Could you check a few things on this model? Use its own coordinates, in mm. Face numbers are marked on the shaded views. A direction names the side the tool comes from. Give positions to 0.01 mm unless a question says otherwise; leave off trailing zeros. Loops run counter-clockwise (first coordinate to the right, second up) from the corner with the lowest first, then second, coordinate; pieces in that order, holes last. Notation, with made-up numbers: (-26, -35) - (15, -35) arc R6 cw to (15, -25) - close; hole circle Ø7 at (2, -0.5). An arc over 180 degrees is marked (long way). Write each question's results on one line, items separated by ' | '. Start each with the question number.
(1) I need wall thicknesses on line 1 (Y direction, x = -5.5, z = 6); line 2 (Y direction, x = 0, z = 12); line 3 (Z direction, x = 14, y = 1). Which ranges of each line are inside material? Lowest first, please.
(2) For pin 1 (12 mm diameter, centred on x = -6.5, y = 17, fed in from +Z); pin 2 (2.5 mm diameter, centred on x = -2.5, z = 12.5, fed in from +Y); pin 3 (1 mm diameter, centred on y = 1.27, z = 1.905, fed in from +X), each with a flat end and sliding along its axis, tell me the tip position at first contact or that it passes through.
(3) Suppose I cut it at D-D (z = 6.5). Please give me the cut outline in (x, y).
(4) If we mould it in two halves opening along X, with no side actions, what happens to the marked faces 1, 2 and 3? For each: released by +X, released by -X, zero draft, split by the parting line, or undercut.
(5) Suppose I cut it at C-C (y = 15). Please give me the cut outline in (x, z) (3 decimals).
(6) Suppose I cut it at A-A (x = 0). Please give me the cut outline in (y, z) (1 decimal), and give its area (3 significant figures).
(7) On a 3-axis mill with a long thin cutter (end or side, diameter ignored), from which of +Z, -Z, +X, -X, +Y, -Y can I reach the whole of each face in a straight line? I mean the marked faces 4, 5, 6 and 7. Say none if no direction works.
(8) Suppose I cut it at B-B (z = 11.5). Please give me the cut outline in (x, y), and give its area (3 significant figures).
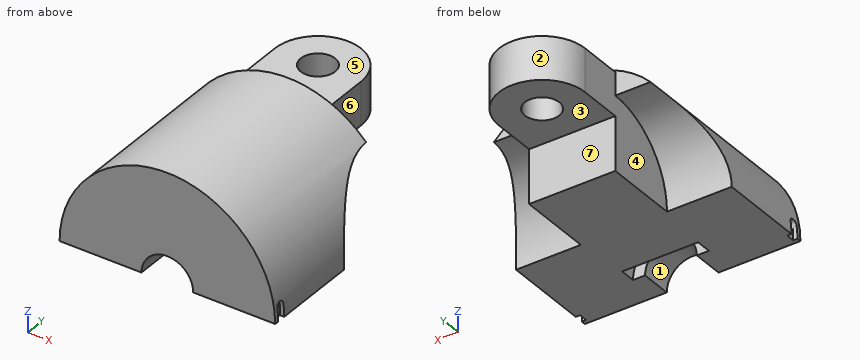
Autodesk Inventor part; units mm, degrees
ref_plane "YZ Plane" through (0, 0, 0) normal (1, 0, 0) x (0, 1, 0)
ref_plane "XZ Plane" through (0, 0, 0) normal (0, 1, 0) x (-1, 0, 0)
ref_plane "XY Plane" through (0, 0, 0) normal (0, 0, 1) x (1, 0, 0)
sketch "Sketch1" plane through (0, 0, 0) normal (0, 1, 0) x (-1, 0, 0)
  arc A0 (15.875, 0) -> (-15.875, 0) centre (0, 0) ccw
  line L0 (15.875, 0) -> (-15.875, 0)
  dimension "d3" = 31.75
extrude "Extrusion1" add sketch "Sketch1" along normal blind 25.4
sketch "Sketch2" plane through (15.875, 0, 0) normal (0, 0, -1) x (-1, 0, 0)
  line L0 (19.685, 0) -> (19.685, 4.572)
  line L1 (19.685, 4.572) -> (21.463, 4.572)
  line L2 (21.463, 4.572) -> (21.463, 6.858)
  line L3 (15.875, 0) -> (15.875, 6.858)
  line L4 (21.463, 6.858) -> (15.875, 6.858)
  line L5 (19.685, 0) -> (15.875, 0)
  line L6 (31.75, 0) -> (0, 0)
  dimension "d12" = 1.778
revolve "Revolution1" cut sketch "Sketch2" angle 360 about axis through (0, 0, 0) along (0, 1, 0)
sketch "Sketch3" plane through (0, 0, 0) normal (1, 0, 0) x (0, 1, 0)
  line L0 (25.4, 0) -> (25.4, 15.875)
  circle A0 centre (25.4, 0) radius 10.9033
  point P0 (0, 0)
extrude "Extrusion2" cut sketch "Sketch3" along normal mid plane 2540
sketch "Sketch4" plane through (0, 25.4, 0) normal (0, 1, 0) x (1, 0, 0)
  line L0 (13.7482, -7.9375) -> (-13.7482, -7.9375)
  line L1 (0, -7.9375) -> (-6.35, -7.9375)
  line L2 (-6.35, -7.9375) -> (-6.35, -14.2875)
  line L3 (-6.35, -14.2875) -> (6.35, -14.2875)
  line L4 (6.35, -14.2875) -> (6.35, -7.9375)
  line L5 (0, -7.9375) -> (6.35, -7.9375)
  line L6 (-6.35, -7.9375) -> (-6.35, 0)
  line L7 (-3.81, 0) -> (-15.875, 0)
  line L8 (-6.35, 0) -> (6.35, 0)
  line L9 (6.35, 0) -> (6.35, -7.9375)
  point P0 (0, 0)
  dimension "d17" = 6.35
  dimension "d18" = 6.35
  dimension "d19" = 12.7
extrude "Extrusion3" add sketch "Sketch4" against normal blind 12.7 contours L0 L6 L7 L8 L9
extrude "Extrusion4" add sketch "Sketch4" along normal blind 2.54 contours L4 L3 L2 L0
sketch "Sketch7" plane through (6.35, 25.4, 7.9375) normal (0, 0, -1) x (-1, 0, 0)
  line L0 (12.7, 0) -> (12.7, 2.54)
  line L1 (0, 0) -> (12.7, 0)
  arc A0 (12.7, 6.35) -> (0, 6.35) centre (6.35, 6.35) ccw
  circle A1 centre (6.35, 6.35) radius 2.54
  line L2 (12.7, 6.35) -> (12.7, 2.54)
  line L3 (12.7, 2.54) -> (0, 2.54)
  line L4 (0, 2.54) -> (0, 6.35)
  point P0 (6.35, -25.4)
  dimension "d31" = 5.08
extrude "Extrusion6" add sketch "Sketch7" against normal blind 6.35
ref_plane "Work Plane1" through (16.51, 17.4625, 0) normal (1, 0, 0) x (0, 0, -1)
sketch "Sketch10" plane through (16.51, 17.4625, 0) normal (1, 0, 0) x (0, 0, -1)
  arc A0 (-1.905, -15.5575) -> (-1.905, -16.8275) centre (-1.905, -16.1925) ccw
  line L0 (-1.905, -15.5575) -> (0, -15.5575)
  line L1 (0, -15.5575) -> (0, -16.8275)
  line L2 (-1.905, -16.8275) -> (0, -16.8275)
  circle A1 centre (-1.905, -16.1925) radius 0.635
extrude "Extrusion7" cut sketch "Sketch10" against normal blind 1.27
extrude "Extrusion8" cut sketch "Sketch10" against normal blind 2.54 contours A1 A0
mirror "Mirror1" about plane through (0, 0, 0) normal (1, 0, 0) of "Extrusion7", "Extrusion8"
sketch "Sketch14" plane through (15.875, 0, 0) normal (0, 0, -1) x (-1, 0, 0)
  line L0 (9.525, 14.4967) -> (9.525, 17.9248)
  line L1 (31.75, 14.4967) -> (22.225, 14.4967)
  line L2 (9.525, 14.4967) -> (22.225, 14.4967)
  line L3 (22.225, 25.4) -> (22.225, 17.9248)
  line L4 (22.225, 14.4967) -> (22.225, 25.4)
  line L5 (9.525, 25.4) -> (22.225, 25.4)
  line L6 (22.225, 25.4) -> (9.525, 25.4)
  line L7 (9.525, 25.4) -> (9.525, 14.4967)
  point P0 (15.875, 0)
extrude "Extrusion9" add sketch "Sketch14" against normal blind 12.7
properties part number "GERMI01-04-01"
Output values:
1) line 1: 0 to 25.4 | line 2: 0 to 29.21, 34.29 to 38.1 | line 3: 0 to 1.33, 2.48 to 7.48
2) pin 1: z = 15.87 | pin 2: y = 37.98 | pin 3: x = 13.97
3) outline: (-14.48, 0) - (14.48, 0) - (14.48, 16.65) - (6.35, 16.65) - (6.35, 25.4) - (-6.35, 25.4) - (-6.35, 16.65) - (-14.48, 16.65) - close
4) face 1: undercut | face 2: split by the parting line | face 3: zero draft
5) outline: (-15.534, 3.274) - (-6.35, 3.274) - (-6.35, 0) - (6.35, 0) - (6.35, 3.274) - (15.534, 3.274) arc R15.875 ccw to start
6) outline: (0, 3.8) - (4.6, 3.8) - (4.6, 5.6) - (6.9, 5.6) - (6.9, 0) - (25.4, 0) - (25.4, 7.9) - (29.2, 7.9) - (29.2, 14.3) - (25.4, 14.3) - (25.4, 15.9) - (0, 15.9) - close; (34.3, 7.9) - (38.1, 7.9) - (38.1, 14.3) - (34.3, 14.3) - close | area: 421 mm2
7) face 4: -Z, -X, +Y | face 5: +Z, +X, -X, +Y | face 6: -Z, +X, +Y | face 7: -Z, +X, -X, +Y
8) outline: (-10.94, 0) - (10.94, 0) - (10.94, 25.4) - (6.35, 25.4) - (6.35, 31.75) arc R6.35 ccw to (-6.35, 31.75) - (-6.35, 25.4) - (-10.94, 25.4) - close; hole circle Ø5.08 at (0, 31.75) | area: 680 mm2
